Verification items for the finished model (mm, model axes). A direction names the side the tool comes from. Coordinates: 2 decimals unless noted, no trailing zeros. Order: outer loops, then holes, each group sorted by start corner. A loop starts at its lowest first (then second) coordinate and runs counter-clockwise, first axis right, second up. Notation, with made-up numbers: (56.5, -10) -> (73.5, -10) arc R13 ccw to (73.5, 2) -> close; hole circle Ø9 at (58, 42). An arc over 180 degrees is marked (long way). Write each question's results on one line, items separated by ' | '. Start each with the question number.
(1) Thickness scan on probe 1 along Y at (x, z) = (-185, 2); probe 2 along Y at (x, z) = (-138.5, -11.5); probe 3 along X at (y, z) = (-11, 0.25). Record the ranges inside material, lowest first. Write a range as [from, to].
(2) Cross-section at B-B on x = -155. Enter the section's corners in (y, z).
(3) Cross-section at C-C on y = -33. Enter the section's corners in (x, z).
(4) Go/stop test with flat-tipped pins: pin 1 (4 mm diameter, centred on y = -40, z = -6.5, fed in from -X); pin 2 (1.5 mm diameter, centred on y = -30.5, z = -9.5, fed in from +X); pin 3 (3.5 mm diameter, centred on x = -84.5, z = 4.5, fed in from -Y). Record where each tip stops, or that it passes through.
(5) Set-up check for faces 1 (the flat face through (-155, -16, 0)), 2 (the flat face through (-161, -30, 3)), 3 (the flat face through (-159, 0, 3)), 4 (the flat face through (-142, -20.901, -9)), 5 (the flat face through (-164.208, -16, -9)): record each of +Z, -Z, +X, -X, +Y, -Y from which the full face is reachable in a straight line by a thin tool's end or side.
(6) Draft check along Y on faces 6 (the flat face through (-133, -32, -7)), 7 (the cylindrical face through (-219.77, -13.5, 3.55)), 8 (the flat face through (-157, -11.761, -1)). Enter one of: +Y half, -Y half, draft (parallel to the pull), parting line (faces both ways), or undercut.
(7) Cross-section at A-A on x = -95. Enter the section's corners in (y, z), and give its area (3 significant figures).
(8) Cross-section at D-D on x = -192. Enter the section's corners in (y, z), and give its area (3 significant figures).
```python
from build123d import *

# Parameters (mm, degrees)
BOSS_EXTRUDE1_DEPTH      = 7
SKETCH2_R                = 5
CUT_EXTRUDE1_DEPTH       = 7
LPATTERN1_COUNT          = 7
LPATTERN1_PITCH          = 30
SKETCH6_R                = 5
CUT_EXTRUDE2_DEPTH       = 10
CUT_EXTRUDE4_REACH       = 219.196
SKETCH9_R                = 1.5
CUT_EXTRUDE9_REACH       = 219.196
SKETCH15_R               = 1.5
SKETCH15_R_2             = 2.5
SKETCH16_W               = 48
SKETCH16_H               = 39.930416712
SKETCH16_R               = 8.2
BOSS_EXTRUDE2_DEPTH      = 15
SKETCH17_W               = 45.833760325
SKETCH17_H               = 30.12512517
SKETCH17_W_2             = 13.763297708
SKETCH17_H_2             = 9.222578979
CUT_EXTRUDE15_DEPTH      = 13
CUT_EXTRUDE16_REACH      = 224.218
SKETCH18_W               = 140
SKETCH18_H               = 115.832892108
FILLET1_R                = 2
BOSS_EXTRUDE4_DEPTH      = 7
CUT_EXTRUDE17_DEPTH      = 10
SKETCH27_W               = 7
SKETCH27_H               = 22
CUT_EXTRUDE18_DEPTH      = 13
CUT_EXTRUDE19_DEPTH      = 266.512692236
CUT_EXTRUDE19_DEPTH_BACK = 266.512692236
SKETCH28_R               = 1.5
CUT_EXTRUDE20_DEPTH      = 266.512692236
CUT_EXTRUDE20_DEPTH_BACK = 266.512692236
SKETCH29_R               = 5


with BuildPart() as part:
    # Sketch1 → Boss-Extrude1 (new body)
    with BuildSketch(Plane.XY):
        with BuildLine():
            Line((-200, 0), (50, 0))
            ThreePointArc((50, 0), (65, -15), (50, -30))
            Line((50, -30), (-200, -30))
            ThreePointArc((-200, -30), (-215, -15), (-200, 0))
        make_face()
    extrude(amount=BOSS_EXTRUDE1_DEPTH)

    # Sketch2 → Cut-Extrude1 (cut)
    with BuildSketch(Plane.XY.offset(7)):
        with Locations((-185, -15)):
            Circle(SKETCH2_R)
    cut_extrude1 = extrude(amount=-CUT_EXTRUDE1_DEPTH, mode=Mode.SUBTRACT)

    # LPattern1: Cut-Extrude1 ×7
    with Locations(*[(i * LPATTERN1_PITCH, 0, 0) for i in range(1, LPATTERN1_COUNT)]):
        add(cut_extrude1, mode=Mode.SUBTRACT)

    # Sketch6 → Cut-Extrude2 (cut)
    with BuildSketch(Plane(origin=(0, 0, 0), x_dir=(-1, 0, 0), z_dir=(0, 0, -1))):
        with Locations((-50, -15)):
            Circle(SKETCH6_R)
    extrude(amount=-CUT_EXTRUDE2_DEPTH, mode=Mode.SUBTRACT)

    # Sketch9 → Cut-Extrude4 (cut, up to next)
    with BuildSketch(Plane(origin=(0, 0, 0), x_dir=(-1, 0, 0), z_dir=(0, 0, -1)), mode=Mode.PRIVATE) as cut_extrude4_sk1:
        with Locations((-29.5, -6.25)):
            Circle(SKETCH9_R)
    cut_extrude4_tool1 = extrude(cut_extrude4_sk1.sketch, amount=-CUT_EXTRUDE4_REACH, mode=Mode.PRIVATE) & part.part
    # Sketch9 → Cut-Extrude4 (cut, up to next)
    with BuildSketch(Plane(origin=(0, 0, 0), x_dir=(-1, 0, 0), z_dir=(0, 0, -1)), mode=Mode.PRIVATE) as cut_extrude4_sk2:
        with Locations((-29.5, -23.75)):
            Circle(SKETCH9_R)
    cut_extrude4_tool2 = extrude(cut_extrude4_sk2.sketch, amount=-CUT_EXTRUDE4_REACH, mode=Mode.PRIVATE) & part.part
    add(cut_extrude4_tool1.solids().sort_by_distance((29.5, -6.25, 0))[0], mode=Mode.SUBTRACT)
    add(cut_extrude4_tool2.solids().sort_by_distance((29.5, -23.75, 0))[0], mode=Mode.SUBTRACT)

    # Sketch15 → Cut-Extrude9 (cut, up to next)
    with BuildSketch(Plane(origin=(0, 0, 0), x_dir=(1, 0, 0), z_dir=(0, 1, 0)), mode=Mode.PRIVATE) as cut_extrude9_sk1:
        with Locations(Location((-195.8, -3.5, 0), (0, 0, 180))):
            Circle(SKETCH15_R)
    cut_extrude9_tool1 = extrude(cut_extrude9_sk1.sketch, amount=-CUT_EXTRUDE9_REACH, mode=Mode.PRIVATE) & part.part
    # Sketch15 → Cut-Extrude9 (cut, up to next)
    with BuildSketch(Plane(origin=(0, 0, 0), x_dir=(1, 0, 0), z_dir=(0, 1, 0)), mode=Mode.PRIVATE) as cut_extrude9_sk2:
        with Locations(Location((45.8, -3.5, 0), (0, 0, 180))):
            Circle(SKETCH15_R_2)
    cut_extrude9_tool2 = extrude(cut_extrude9_sk2.sketch, amount=-CUT_EXTRUDE9_REACH, mode=Mode.PRIVATE) & part.part
    add(cut_extrude9_tool1.solids().sort_by_distance((-195.8, 0, 3.5))[0], mode=Mode.SUBTRACT)
    add(cut_extrude9_tool2.solids().sort_by_distance((45.8, 0, 3.5))[0], mode=Mode.SUBTRACT)

    # Sketch16 → Boss-Extrude2 (add)
    with BuildSketch(Plane(origin=(0, 0, 0), x_dir=(-1, 0, 0), z_dir=(0, 0, -1))):
        with Locations((157, -31.726084321)):
            Rectangle(SKETCH16_W, SKETCH16_H)
        with Locations((144.145834, -39.243444981)):
            Circle(SKETCH16_R, mode=Mode.SUBTRACT)
        with Locations((170.306394211, -39.243444981)):
            Circle(SKETCH16_R, mode=Mode.SUBTRACT)
        with BuildLine():
            Line((153.043612384, -45.175236858), (161.648055614, -45.175236858))
            ThreePointArc((161.648055614, -45.175236858), (163.390378659, -46.917559902), (161.648055614, -48.659882947))
            Line((161.648055614, -48.659882947), (153.043612384, -48.659882947))
            ThreePointArc((153.043612384, -48.659882947), (151.301289339, -46.917559902), (153.043612384, -45.175236858))
        make_face(mode=Mode.SUBTRACT)
    extrude(amount=BOSS_EXTRUDE2_DEPTH)

    # Sketch17 → Cut-Extrude15 (cut)
    with BuildSketch(Plane(origin=(0, 0, -15), x_dir=(-1, 0, 0), z_dir=(0, 0, -1))):
        with Locations((156.666880163, -35.963336462)):
            Rectangle(SKETCH17_W, SKETCH17_H)
        with Locations((157.326506844, -16.372165454)):
            Rectangle(SKETCH17_W_2, SKETCH17_H_2)
    extrude(amount=-CUT_EXTRUDE15_DEPTH, mode=Mode.SUBTRACT)

    # Sketch18 → Cut-Extrude16 (cut, up to next)
    with BuildSketch(Plane.XY.offset(7), mode=Mode.PRIVATE) as cut_extrude16_sk1:
        with Locations((-5, -15.036727437)):
            Rectangle(SKETCH18_W, SKETCH18_H)
    cut_extrude16_tool1 = extrude(cut_extrude16_sk1.sketch, amount=-CUT_EXTRUDE16_REACH, mode=Mode.PRIVATE) & part.part
    add(cut_extrude16_tool1.solids().sort_by_distance((-5, -15.036727, 7))[0], mode=Mode.SUBTRACT)

    # Fillet1
    # the kernel refuses this fillet: 2 mm, written as the material it takes off along each edge
    with BuildSketch(Plane(origin=(-133, -51.691292677, 5), x_dir=(0, 1, 0), z_dir=(0, 0, -1))) as fillet1_piece_1:
        with BuildLine():
            CenterArc((FILLET1_R, -FILLET1_R), FILLET1_R, 90, 90)
            Line((0, -FILLET1_R), (0, 0))
            Line((0, 0), (FILLET1_R, 0))
        make_face()
    extrude(amount=25, mode=Mode.SUBTRACT)
    with BuildSketch(Plane(origin=(-181, -51.691292677, 5), x_dir=(0, 1, 0), z_dir=(0, 0, -1))) as fillet1_piece_2:
        with BuildLine():
            CenterArc((FILLET1_R, FILLET1_R), FILLET1_R, 180, 90)
            Line((0, FILLET1_R), (0, 0))
            Line((0, 0), (FILLET1_R, 0))
        make_face()
    extrude(amount=25, mode=Mode.SUBTRACT)
    with BuildSketch(Plane(origin=(-181, -11.760875965, 0), x_dir=(0, -1, 0), z_dir=(0, 0, -1)), Plane(origin=(-133, -11.760875965, 0), x_dir=(-1, 0, 0), z_dir=(0, 0, -1))) as fillet1_piece_3:
        with BuildLine():
            CenterArc((FILLET1_R, -FILLET1_R), FILLET1_R, 90, 90)
            Line((0, -FILLET1_R), (0, 0))
            Line((0, 0), (FILLET1_R, 0))
        make_face()
    extrude(amount=20, mode=Mode.SUBTRACT)

    # Sketch24 → Boss-Extrude4 (add)
    with BuildSketch(Plane(origin=(0, 0, 0), x_dir=(-1, 0, 0), z_dir=(0, 0, -1))):
        with BuildLine():
            ThreePointArc((245, 0), (260, -15), (245, -30))
            Line((245, -30), (245, 0))
        make_face()
        with BuildLine():
            Line((245, 0), (245, -30))
            Line((245, -30), (200, -30))
            ThreePointArc((200, -30), (215, -15), (200, 0))
            Line((200, 0), (245, 0))
        make_face()
    extrude(amount=-BOSS_EXTRUDE4_DEPTH)

    # Sketch25 → Cut-Extrude17 (cut)
    with BuildSketch(Plane(origin=(0, 0, 0), x_dir=(-1, 0, 0), z_dir=(0, 0, -1))):
        with BuildLine():
            ThreePointArc((237.45, -25), (237.010660172, -23.939339828), (235.95, -23.5))
            Line((235.95, -23.5), (235.95, -26.5))
            ThreePointArc((235.95, -26.5), (237.010660172, -26.060660172), (237.45, -25))
        make_face()
        with BuildLine():
            Line((235.95, -26.5), (235.95, -23.5))
            ThreePointArc((235.95, -23.5), (234.45, -25), (235.95, -26.5))
        make_face()
        with BuildLine():
            ThreePointArc((237.45, -5), (237.010660172, -3.939339828), (235.95, -3.5))
            Line((235.95, -3.5), (235.95, -6.5))
            ThreePointArc((235.95, -6.5), (237.010660172, -6.060660172), (237.45, -5))
        make_face()
        with BuildLine():
            Line((235.95, -6.5), (235.95, -3.5))
            ThreePointArc((235.95, -3.5), (234.45, -5), (235.95, -6.5))
        make_face()
    extrude(amount=-CUT_EXTRUDE17_DEPTH, mode=Mode.SUBTRACT)

    # Sketch27 → Cut-Extrude18 (cut)
    with BuildSketch(Plane(origin=(-75, 0, 0), x_dir=(0, 0, -1), z_dir=(1, 0, 0))):
        with Locations((-3.5, -15)):
            Rectangle(SKETCH27_W, SKETCH27_H)
    extrude(amount=-CUT_EXTRUDE18_DEPTH, mode=Mode.SUBTRACT)

    # Sketch28 → Cut-Extrude19 (cut, two sides: drawn at the far end of the back side and taken through both)
    with BuildSketch(Plane(origin=(0, 0, 0), x_dir=(1, 0, 0), z_dir=(0, 1, 0)).offset(-CUT_EXTRUDE19_DEPTH_BACK)):
        with Locations(Location((-82, -3.5, 0), (0, 0, 180))):
            Circle(SKETCH28_R)
    extrude(amount=CUT_EXTRUDE19_DEPTH + CUT_EXTRUDE19_DEPTH_BACK, mode=Mode.SUBTRACT)

    # Sketch29 → Cut-Extrude20 (cut, two sides: drawn at the far end of the back side and taken through both)
    with BuildSketch(Plane(origin=(0, 0, 0), x_dir=(-1, 0, 0), z_dir=(0, 0, -1)).offset(-CUT_EXTRUDE20_DEPTH_BACK)):
        with Locations((215, -15)):
            Circle(SKETCH29_R)
    extrude(amount=CUT_EXTRUDE20_DEPTH + CUT_EXTRUDE20_DEPTH_BACK, mode=Mode.SUBTRACT)


solid = part.part
```
Results are:
1) probe 1: y = [-30, -20], [-10, 0] | probe 2: y = [-51.69, -51.03], [-20.9, -11.76] | probe 3: x = [-259.46, -218], [-212, -188], [-182, -158], [-152, -128], [-122, -98], [-92, -88]
2) outline: (-51.69, -15) -> (-51.03, -15) -> (-51.03, -2) -> (-48.66, -2) -> (-48.66, 0) -> (-51.69, 0) -> close; (-45.18, -2) -> (-11.76, -2) -> (-11.76, 0) -> (-20, 0) -> (-20, 7) -> (-30, 7) -> (-30, 0) -> (-45.18, 0) -> close; (-10, 0) -> (0, 0) -> (0, 7) -> (-10, 7) -> close
3) outline: (-181, -15) -> (-179.58, -15) -> (-179.58, -2) -> (-175.62, -2) -> (-175.62, 0) -> (-181, 0) -> close; (-164.99, -2) -> (-149.46, -2) -> (-149.46, 0) -> (-164.99, 0) -> close; (-138.83, -2) -> (-133.75, -2) -> (-133.75, -15) -> (-133, -15) -> (-133, 0) -> (-138.83, 0) -> close
4) pin 1: stops at x = -181 | pin 2: stops at x = -133 | pin 3: stops at y = -30
5) face 1: +Z | face 2: +Z, +X, -X, -Y | face 3: +Z, -Z, +X, -X, +Y | face 4: -Z | face 5: -Z, +Y
6) face 6: draft | face 7: undercut | face 8: +Y half
7) outline: (-30, 0) -> (-20, 0) -> (-20, 7) -> (-30, 7) -> close; (-10, 0) -> (0, 0) -> (0, 7) -> (-10, 7) -> close | area: 140 mm2
8) outline: (-30, 0) -> (0, 0) -> (0, 7) -> (-30, 7) -> close | area: 210 mm2
